```python
from build123d import *

# Parameters (mm, degrees)
F0_R     = 31.75
F1_DEPTH = 19.05
F2_R     = 26.67
F4_DEPTH = 5.08
F3_R     = 26.67
F5_DEPTH = 5.08
F6_R     = 7.874
F7_DEPTH = 50.8


with BuildPart() as f1:
    # F0 (on Top) → F1 (new body, symmetric)
    with BuildSketch(Plane.XY):
        Circle(F0_R)
    extrude(amount=F1_DEPTH, both=True)

    # F2 (on face) → F4 (cut)
    with BuildSketch(Plane.XY.offset(19.05)):
        Circle(F2_R)
    extrude(amount=-F4_DEPTH, mode=Mode.SUBTRACT)

    # F3 (on face) → F5 (cut)
    with BuildSketch(Plane(origin=(0, 0, -19.05), x_dir=(1, 0, 0), z_dir=(0, 0, -1))):
        Circle(F3_R)
    extrude(amount=-F5_DEPTH, mode=Mode.SUBTRACT)

    # F6 (on face) → F7 (cut)
    with BuildSketch(Plane.XY.offset(13.97)):
        Circle(F6_R)
    extrude(amount=-F7_DEPTH, mode=Mode.SUBTRACT)


solid = f1.part
```
Verification items for the finished model (mm, model axes). A direction names the side the tool comes from. Round coordinates to 2 decimals unless told otherwise and drop trailing zeros. Write each loop counter-clockwise with the first axis right and the second up, starting at its lowest first coordinate (ties: lowest second). Pieces come first, ordered by that corner, then holes. Notation, with made-up numbers: (10.5, 30.25) -> (67.5, 30.25) arc R17 ccw to (67.5, 41.25) -> close; hole circle Ø6 at (16, 20.5). An arc over 180 degrees is marked (long way). Write each question's results on one line, items separated by ' | '. Start each with the question number.
1. Cross-section at A-A (y = 0). Enter the section's corners in (x, z), then the cut area to 3 significant figures.
2. Draft check along X on faces 1 (the flat face through (-7, 26, 19.05)), 2 (the cylindrical face through (-1.707, -7.687, 0.196)), 3 (the cylindrical face through (-6.883, -30.995, 0.267)). Enter one of: +X half, -X half, draft (parallel to the pull), parting line (faces both ways), or undercut.
3. Cross-section at C-C (z = -16). Enter the section's corners in (x, y), then the cut area to 3 significant figures.
4. Set-up check for faces 4 (the flat face through (-7, 26, -19.05)), 5 (the flat face through (-6, 6, -13.97)), 6 (the flat face through (-6, -6, 13.97)): record each of +Z, -Z, +X, -X, +Y, -Y from which the full face is reachable in a straight line by a thin tool's end or side.
5. Depth check by flat-ended pin: P1, Ø2, axis at x = 2, y = 9.5, coming from the -Z side; P2, Ø10, axis at x = -1.5, z = -14, coming from the +Y side; P3, Ø6, axis at x = 3, z = 14.5, coming from the -Y side. Enter the tip coordinate at first touch or a pass-through.
6. Cross-section at D-D (x = -21.5). Enter the section's corners in (y, z).
7. Material ranges on probe 1 along Y at (x, z) = (0, 17.25); probe 2 along Y at (x, z) = (0, -1.75); probe 3 along Z at (x, y) = (-16, -9), recorded low to high. Write a range as from..to.
Solutions:
1) outline: (-31.75, -19.05) -> (-26.67, -19.05) -> (-26.67, -13.97) -> (-7.87, -13.97) -> (-7.87, 13.97) -> (-26.67, 13.97) -> (-26.67, 19.05) -> (-31.75, 19.05) -> close; (7.87, -13.97) -> (26.67, -13.97) -> (26.67, -19.05) -> (31.75, -19.05) -> (31.75, 19.05) -> (26.67, 19.05) -> (26.67, 13.97) -> (7.87, 13.97) -> close | area: 1,440 mm2
2) face 1: draft | face 2: undercut | face 3: parting line
3) outline: circle Ø63.5 at (0, 0); hole circle Ø53.34 at (0, 0) | area: 932 mm2
4) face 4: -Z, +X, -X, +Y, -Y | face 5: -Z | face 6: +Z
5) P1: stops at z = -13.97 | P2: stops at y = 31.75 | P3: stops at y = -31.75
6) outline: (-23.36, -19.05) -> (-15.78, -19.05) -> (-15.78, -13.97) -> (15.78, -13.97) -> (15.78, -19.05) -> (23.36, -19.05) -> (23.36, 19.05) -> (15.78, 19.05) -> (15.78, 13.97) -> (-15.78, 13.97) -> (-15.78, 19.05) -> (-23.36, 19.05) -> close
7) probe 1: y = -31.75..-26.67, 26.67..31.75 | probe 2: y = -31.75..-7.87, 7.87..31.75 | probe 3: z = -13.97..13.97
